Input: part model. Units: mm. Frame: model coordinates. A direction names the side the tool comes from. Coordinates: 2 decimals unless noted, no trailing zeros. Loops run counter-clockwise (first coordinate to the right, second up) from the corner with the lowest first, then second, coordinate; pieces in that order, holes last. Notation, with made-up numbers: (83.25, 9) -> (102.25, 9) arc R19 cw to (102.25, 25) -> close; hole circle Ø5 at (86.5, -29.5). An arc over 180 degrees is marked (long way). Put each result on its own line as item: value. Start each with the question number.
1) Contact query for flat-ended pins moving along their axis: P1, Ø1.5, axis at x = -1, z = 7, coming from the -Y side; P2, Ø2.5, axis at y = 1, z = 4.5, coming from the +X side; P3, Ø4, axis at x = 0.5, z = 24.5, coming from the +Y side. Output: stop coordinate, or through.
2) Cut plane B-B (y = 0). Return the cut outline in (x, z), plus the area to 3 significant figures.
3) Cut plane A-A (x = 3.5). Return the cut outline in (y, z), plus the area to 3 significant figures.
4) Cut plane D-D (x = 0). Return the cut outline in (y, z).
5) Material intervals for L1, parallel to X at y = 0.25, z = 37; L2, parallel to Z at x = 3.5, y = 2.5; L3, parallel to Y at x = -3, z = 16.5, sorted ascending.
6) Set-up query: faces 1 (the flat face through (3, 0, 32)), 2 (the flat face through (-3, -3, 22)), 3 (the flat face through (-3, -3, 18)), 4 (the flat face through (0, 0, 50)). Return all of +Z, -Z, +X, -X, +Y, -Y with unobstructed straight access to the full face (end or side cutting, diameter ignored); none if empty.
7) Cut plane C-C (z = 31). Return the cut outline in (x, y).
from build123d import *

# Parameters (mm, degrees)
SKETCH_1_R          = 4
EXTRUDE_1_DEPTH     = 18
SKETCH_2_R          = 4.5
EXTRUDE_2_DEPTH     = 4
SKETCH_3_R          = 4
EXTRUDE_3_DEPTH     = 28
SKETCH_4_W          = 6
SKETCH_4_H          = 6
CUT_EXTRUDE_1_DEPTH = 1
SKETCH_5_W          = 6
SKETCH_5_H          = 6
CUT_EXTRUDE_2_DEPTH = 1


with BuildPart() as part:
    # 草圖1 → 填料-伸長1 (new body)
    with BuildSketch(Plane.XY):
        Circle(SKETCH_1_R)
    extrude(amount=EXTRUDE_1_DEPTH)

    # 草圖2 → 填料-伸長2 (add)
    with BuildSketch(Plane.XY.offset(18)):
        Circle(SKETCH_2_R)
    extrude(amount=EXTRUDE_2_DEPTH)

    # 草圖3 → 填料-伸長3 (add)
    with BuildSketch(Plane.XY.offset(22)):
        Circle(SKETCH_3_R)
    extrude(amount=EXTRUDE_3_DEPTH)

    # 草圖4 → 除料-伸長1 (cut)
    with BuildSketch(Plane(origin=(4, 0, 0), x_dir=(0, 0, -1), z_dir=(1, 0, 0))):
        with Locations((-32, 0)):
            Rectangle(SKETCH_4_W, SKETCH_4_H)
    extrude(amount=-CUT_EXTRUDE_1_DEPTH, mode=Mode.SUBTRACT)

    # 草圖5 → 除料-伸長2 (cut)
    with BuildSketch(Plane(origin=(4, 0, 0), x_dir=(0, 0, -1), z_dir=(1, 0, 0))):
        with Locations((-4, 0)):
            Rectangle(SKETCH_5_W, SKETCH_5_H)
    extrude(amount=-CUT_EXTRUDE_2_DEPTH, mode=Mode.SUBTRACT)


solid = part.part
Results found:
1. P1: stops at y = -3.99
1. P2: stops at x = 3
1. P3: stops at y = 4
2. outline: (-4.5, 18) -> (-4, 18) -> (-4, 0) -> (4, 0) -> (4, 1) -> (3, 1) -> (3, 7) -> (4, 7) -> (4, 18) -> (4.5, 18) -> (4.5, 22) -> (4, 22) -> (4, 29) -> (3, 29) -> (3, 35) -> (4, 35) -> (4, 50) -> (-4, 50) -> (-4, 22) -> (-4.5, 22) -> close
2. area: 392 mm2
3. outline: (-2.83, 18) -> (-1.94, 18) -> (-1.94, 7) -> (1.94, 7) -> (1.94, 18) -> (2.83, 18) -> (2.83, 22) -> (1.94, 22) -> (1.94, 29) -> (-1.94, 29) -> (-1.94, 22) -> (-2.83, 22) -> close; (-1.94, 0) -> (1.94, 0) -> (1.94, 1) -> (-1.94, 1) -> close; (-1.94, 35) -> (1.94, 35) -> (1.94, 50) -> (-1.94, 50) -> close
3. area: 154 mm2
4. outline: (-4.5, 18) -> (-4, 18) -> (-4, 0) -> (4, 0) -> (4, 18) -> (4.5, 18) -> (4.5, 22) -> (4, 22) -> (4, 50) -> (-4, 50) -> (-4, 22) -> (-4.5, 22) -> close
5. L1: x = -3.99 to 3.99
5. L2: z = 18 to 22
5. L3: y = -2.65 to 2.65
6. face 1: +X, +Y, -Y
6. face 2: +Z
6. face 3: -Z
6. face 4: +Z, +X, -X, +Y, -Y
7. outline: (3, -2.65) -> (3, 2.65) arc R4 ccw (long way) to start
